Can you work these out from the drawing? Everything is in mm from the part's minimum corner. A direction names the side the tool comes from. Round coordinates to 2 decimals unless told otherwise and drop trailing zeros. Loops run counter-clockwise (first coordinate to the right, second up) from the corner with the lowest first, then second, coordinate; pieces in that order, holes last. Notation, with made-up numbers: M 4.25,-27.75 L 56.25,-27.75 A26 ccw 56.25,3.25 Z; hole C -19.75,71.5 d11. An arc over 180 degrees is marked long. Use a Markdown table: item, result.
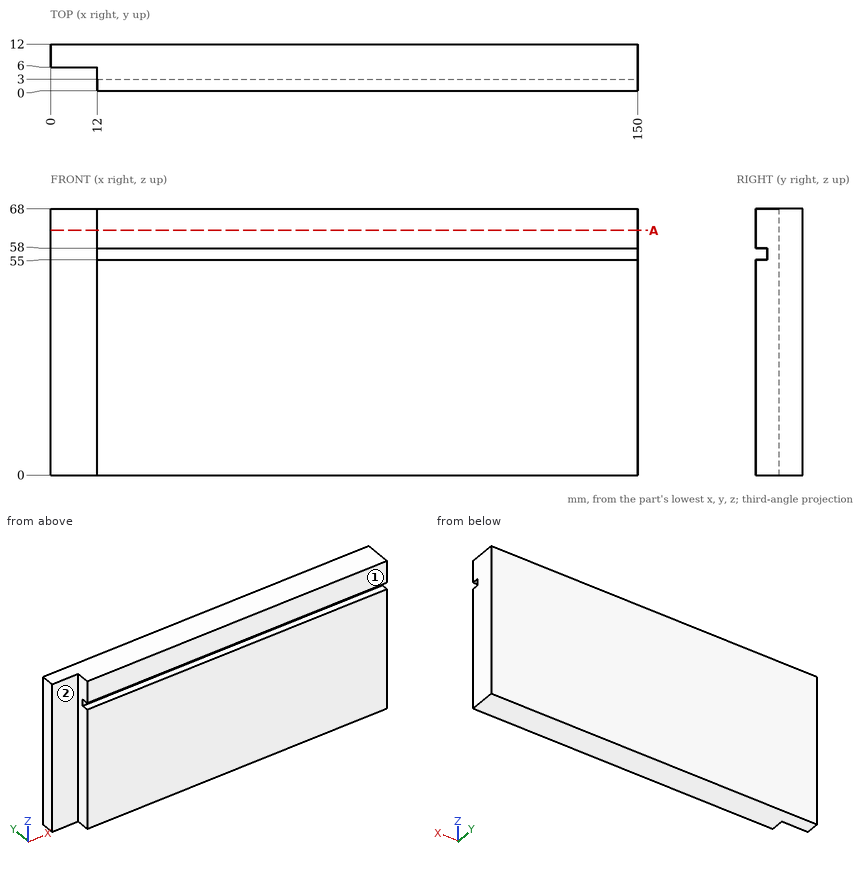
1. I need wall thicknesses on probe 1 along Z at (x, y) = (97.5, 1.5); probe 2 along X at (y, z) = (2, 41.5). Which ranges of each line are inside material? Lowest first, please. Write a range as from..to.
Answer sheet:
| item | result |
|---|---|
| probe 1 | 0..55, 58..68 |
| probe 2 | 12..150 |
2. For pin 1 Ø1 at (y, z) = (3.5, 53) entering from -X, with a flat end and sliding along its axis, tell me the tip position at first contact or that it passes through.
Answer sheet:
| item | result |
|---|---|
| pin 1 | x = 12 |
3. Which directions (+Z, -Z, +X, -X, +Y, -Y) give clear straight access to the entire face, cutting with the end or side of a thin tool? Please do the marked faces 1 and 2.
Answer sheet:
| item | result |
|---|---|
| face 1 | +Z, -Z, +X, -X, -Y |
| face 2 | +Z, -Z, -X, -Y |
4. Imagine slicing it at A-A, the plane z = 62.5. Write out the boundary of the cut face in (x, y).
Answer sheet:
| item | result |
|---|---|
| outline | M 0,6 L 12,6 L 12,0 L 150,0 L 150,12 L 0,12 Z |
